Input: part model. Units: mm. Frame: model coordinates. Face numbers are marked on the shaded views. A direction names the side the tool comes from. Coordinates: 2 decimals unless noted, no trailing zeros. Order: outer loops, then holes, each group sorted by start corner. A loop starts at its lowest first (then second) coordinate and runs counter-clockwise, first axis right, second up. Notation, with made-up numbers: M 53.5,-34.75 L 61.5,-34.75 A35 ccw 61.5,-0.75 Z; hole C 52,36.25 d2. An arc over 180 degrees is marked long. Answer in a Markdown table with one row per item.
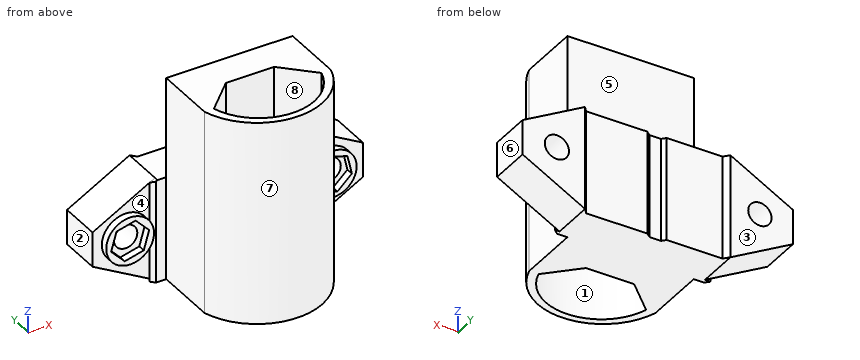
from build123d import *

# Parameters (mm, degrees)
F1_DEPTH  = 20.32
F3_DEPTH  = 53.848
F5_DEPTH  = 25.4
F7_DEPTH  = 54.356
F8_R      = 11.508682
F8_R_2    = 11.649308
F9_DEPTH  = 3.556
F10_R     = 5.689176
F10_R_2   = 5.902235
F11_DEPTH = 29.972
F13_DEPTH = 99.568
F14_W     = 23.597419
F14_H     = 13.089193
F14_H_2   = 14.010968
F15_DEPTH = 18.034
F17_DEPTH = 99.568


with BuildPart() as f1:
    # F0 (on Front) → F1 (new body)
    with BuildSketch(Plane.XZ):
        Polygon((0, 0), (-70.953442, 0), (-101.433442, -16.739016), (-101.433442, -33.727869), (-70.953442, -50.466886), (0, -50.466886), (30.48, -33.727869), (30.48, -16.739016), align=None)
    extrude(amount=F1_DEPTH)

    # F2 (on face) → F3 (join)
    with BuildSketch(Plane(origin=(0, 0, -50.466886), x_dir=(1, 0, 0), z_dir=(0, 0, -1))):
        Polygon((-73.638171, 20.32), (2.316022, 20.279033), (0, 22.306934), (-71.794622, 22.306934), align=None)
    extrude(amount=-F3_DEPTH)

    # F4 (on face) → F5 (cut)
    with BuildSketch(Plane(origin=(0.010938, -20.280276, 0), x_dir=(-1, -0.000539, 0), z_dir=(-0.000539, 1, 0))):
        Polygon((70.964391, 0), (73.64912, -1.4744), (73.64912, 3.381114), (-2.305084, 3.381114), (-2.305084, -1.271914), (0.010938, 0), align=None)
    extrude(amount=-F5_DEPTH, mode=Mode.SUBTRACT)

    # F6 (on face) → F7 (cut)
    with BuildSketch(Plane.XY):
        Polygon((-2.108495, -2.580968), (0, 0), (-70.953442, 0), (-68.660595, -2.580968), (-41.376077, -2.580968), (-39.716881, -4.424516), (-34.186237, -4.424516), (-31.973977, -2.580968), align=None)
    extrude(amount=-F7_DEPTH, mode=Mode.SUBTRACT)

    # F8 (on face) → F9 (join)
    with BuildSketch(Plane.XZ.offset(20.32)):
        with Locations((13.702015, -24.732648)):
            Circle(F8_R)
        Polygon((4.514804, -21.914458), (11.549033, -15.367195), (20.736244, -18.185385), (22.889225, -27.550837), (15.854996, -34.0981), (6.667786, -31.279911), align=None, mode=Mode.SUBTRACT)
        with Locations((-85.277705, -24.443241)):
            Circle(F8_R_2)
        Polygon((-94.556486, -26.755789), (-91.919821, -17.563855), (-82.641039, -15.251307), (-75.998923, -22.130693), (-78.635589, -31.322628), (-87.91437, -33.635176), align=None, mode=Mode.SUBTRACT)
    extrude(amount=F9_DEPTH)

    # F10 (on face) → F11 (cut)
    with BuildSketch(Plane.XZ.offset(20.32)):
        with Locations((-85.302033, -24.321858)):
            Circle(F10_R)
        with Locations((13.746024, -24.519194)):
            Circle(F10_R_2)
    extrude(amount=-F11_DEPTH, mode=Mode.SUBTRACT)

    # F12 (on face) → F13 (join)
    with BuildSketch(Plane(origin=(0, 0, -50.466886), x_dir=(1, 0, 0), z_dir=(0, 0, -1))):
        Polygon((-66.714622, 52.786934), (-66.714622, 22.306934), (-5.08, 22.306934), (-5.08, 52.786934), (-9.652, 52.786934), (-23.981169, 38.53016), (-47.578588, 38.53016), (-62.142622, 52.786934), align=None)
    extrude(amount=-F13_DEPTH)

    # F14 (on face) → F15 (cut)
    with BuildSketch(Plane.XZ.offset(38.53016)):
        with Locations((-35.779878, -35.672662)):
            Rectangle(F14_W, F14_H)
        with Locations((-35.779878, -14.010968)):
            Rectangle(F14_W, F14_H_2)
    extrude(amount=-F15_DEPTH, mode=Mode.SUBTRACT)

    # F16 (on face) → F17 (join)
    with BuildSketch(Plane(origin=(0, 0, -50.466886), x_dir=(1, 0, 0), z_dir=(0, 0, -1))):
        with BuildLine():
            Line((-9.652, 52.786934), (-5.08, 52.786934))
            ThreePointArc((-5.08, 52.786934), (-35.897311, 76.1177), (-66.714622, 52.786934))
            Line((-66.714622, 52.786934), (-62.142622, 52.786934))
            ThreePointArc((-62.142622, 52.786934), (-35.897311, 72.694804), (-9.652, 52.786934))
        make_face()
    extrude(amount=-F17_DEPTH)


solid = f1.part
1) Mould query, pull axis X, two halves, no side actions, for the marked faces 1, 2 and 3. Classes: +X half, -X half, draft (parallel to the pull), parting line (faces both ways), or undercut.
Resolved:
| item | result |
|---|---|
| face 1 | undercut |
| face 2 | -X half |
| face 3 | draft |
2) Cut plane A-A, the plane z = 3. Output: boundary loops of the cut face in (x, y).
Resolved:
| item | result |
|---|---|
| outline | M -66.71,-52.79 A32.02 ccw -5.08,-52.79 L -5.08,-22.31 L -66.71,-22.31 Z; hole M -62.14,-52.79 A27.25 ccw -9.65,-52.79 L -23.98,-38.53 L -47.58,-38.53 Z |
3) Cut plane C-C, the plane x = -60. Output: boundary loops of the cut face in (y, z), and give its area (3 significant figures).
Resolved:
| item | result |
|---|---|
| outline | M -65.18,-50.47 L -58.16,-50.47 L -58.16,49.1 L -65.18,49.1 Z; M -50.69,-50.47 L -2.58,-50.47 L -2.58,0 L -22.31,0 L -22.31,49.1 L -50.69,49.1 Z |
| area | 4,520 mm2 |
4) Contact query for flat-ended pins moving along their axis: pin 1 (14.5 mm diameter, centred on y = -32, z = -37, fed in from +X); pin 2 (12 mm diameter, centred on y = -54.5, z = -18, fed in from -X); pin 3 (9 mm diameter, centred on x = 10, z = -21.5, fed in from -Y). Output: stop coordinate, or through.
Resolved:
| item | result |
|---|---|
| pin 1 | stops at x = -5.08 |
| pin 2 | stops at x = -66.71 |
| pin 3 | stops at y = -23.88 |
5) Reachability of the marked faces 4, 5, 6, 7 and 8 from +Z, -Z, +X, -X, +Y, -Y: full face, straight path, thin tool, end or side. Return the list, or none.
Resolved:
| item | result |
|---|---|
| face 4 | -Y |
| face 5 | +Z, +X, -X, +Y |
| face 6 | +Z, -Z, +X, +Y, -Y |
| face 7 | +Z, -Z, -Y |
| face 8 | +Z, -Z |
6) Cut plane B-B, the plane y = -28.5. Output: boundary loops of the cut face in (x, z).
Resolved:
| item | result |
|---|---|
| outline | M -66.71,-50.47 L -5.08,-50.47 L -5.08,49.1 L -66.71,49.1 Z; hole M -47.58,-42.22 L -23.98,-42.22 L -23.98,-29.13 L -47.58,-29.13 Z; hole M -47.58,-21.02 L -23.98,-21.02 L -23.98,-7.01 L -47.58,-7.01 Z |
7) Cut plane D-D, the plane y = -70.5. Output: boundary loops of the cut face in (x, z).
Resolved:
| item | result |
|---|---|
| outline | M -54.01,-50.47 L -46.61,-50.47 L -46.61,49.1 L -54.01,49.1 Z; M -25.18,-50.47 L -17.78,-50.47 L -17.78,49.1 L -25.18,49.1 Z |
8) Material intervals for probe 1 along Z at (x, y) = (-61, -3.5); probe 2 along X at (y, z) = (-25.5, 30.5); probe 3 along X at (y, z) = (-26, -10.5), sorted ascending.
Resolved:
| item | result |
|---|---|
| probe 1 | z = -50.47 to 0 |
| probe 2 | x = -66.71 to -5.08 |
| probe 3 | x = -66.71 to -47.58, -23.98 to -5.08 |
